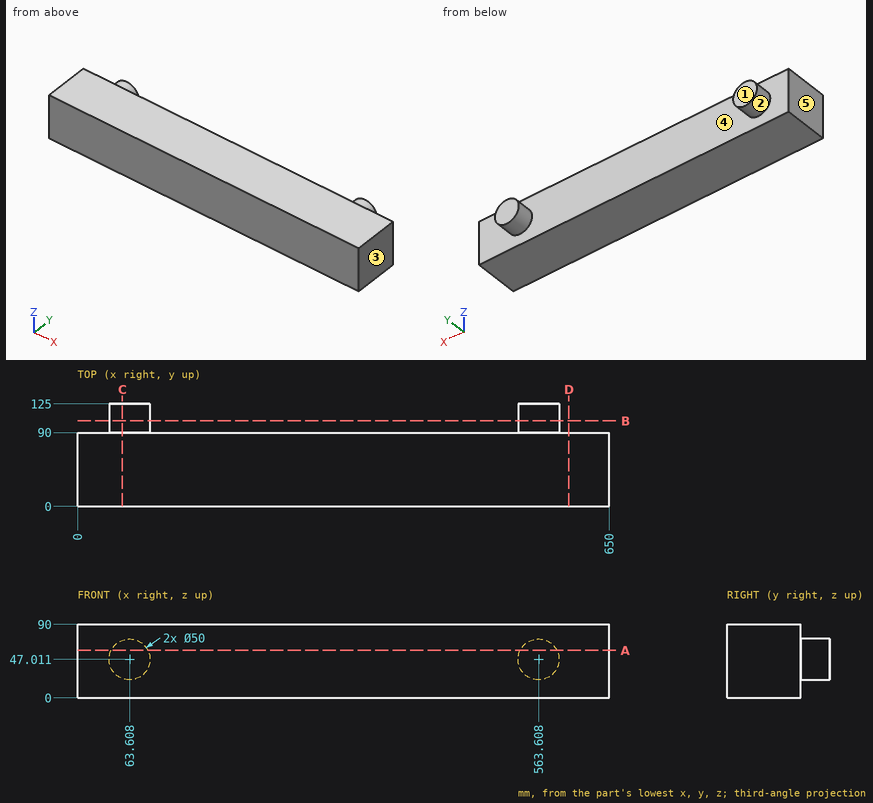
Verification items for this drawing (mm, ordinates from the low corner). A direction names the side the tool comes from. Round coordinates to 2 decimals unless told otherwise and drop trailing zeros. Order: outer loops, then holes, each group sorted by start corner. A loop starts at its lowest first (then second) coordinate and runs counter-clockwise, first axis right, second up. Notation, with made-up numbers: (84.5, 20.5) - (128.5, 20.5) arc R7 ccw to (128.5, 29.5) - close; hole circle Ø10 at (84, -34.5). An arc over 180 degrees is marked (long way). Use CSV: the item, a comma, the result in double quotes.
(1) Section check D-D on x = 600.5. Record the boundary of the cut face in (y, z), and give its area (3 significant figures).
Entries:
outline,"(0, 0) - (90, 0) - (90, 90) - (0, 90) - close"
area,"8,100 mm^2"
(2) Access from +Z, -Z, +X, -X, +Y, -Y to the whole of each face (thin tool, end or side, straight path). Record for the marked faces 1 and 2.
Entries:
face 1,"+Z, -Z, +X, -X, +Y"
face 2,"+Y"
(3) Section check A-A on z = 58. Record the boundary of the cut face in (x, y).
Entries:
outline,"(0, 0) - (650, 0) - (650, 90) - (586.06, 90) - (586.06, 125) - (541.15, 125) - (541.15, 90) - (86.06, 90) - (86.06, 125) - (41.15, 125) - (41.15, 90) - (0, 90) - close"
(4) Section check B-B on y = 104.5. Record the boundary of the cut face in (x, z), and give its area (3 significant figures).
Entries:
outline,"circle Ø50 at (63.61, 47.01); circle Ø50 at (563.61, 47.01)"
area,"3,930 mm^2"
(5) Gauge pin test, flat ends, axial feed: pin 1 Ø2 at (x, z) = (269, 15) entering from +Y; pin 2 Ø3 at (y, z) = (103.5, 58) entering from -X. Record the tip position at first contact, or that the pin passes through.
Entries:
pin 1,"y = 90"
pin 2,"x = 40.48"
(6) Mould release check, pull along X, two halves, no side actions. Record for the marked faces 3, 4 and 5: released by +X, released by -X, zero draft, split by the parting line, or undercut.
Entries:
face 3,"released by +X"
face 4,"undercut"
face 5,"released by -X"
(7) Section check C-C on x = 55. Record the boundary of the cut face in (y, z).
Entries:
outline,"(0, 0) - (90, 0) - (90, 23.54) - (125, 23.54) - (125, 70.48) - (90, 70.48) - (90, 90) - (0, 90) - close"
(8) Thickness scan on probe 1 along Y at (x, z) = (194.5, 81.5); probe 2 along Z at (x, y) = (74.5, 115) (1 decimal). Record the ranges inside material, lowest first. Write a range as from..to.
Entries:
probe 1,"0..90"
probe 2,"24.5..69.5"
